The model under review builds one solid part; all positions refer to its coordinate system, in mm. Face numbers are marked on the shaded views. A direction names the side the tool comes from. Coordinates: 2 decimals unless noted, no trailing zeros. Write each loop counter-clockwise with the first axis right and the second up, starting at its lowest first coordinate (ties: lowest second). Pieces come first, ordered by that corner, then holes. Notation, with made-up numbers: M -10.75,-2.75 L 40.25,-2.75 A15 cw 40.25,6.25 Z; hole C 8,62 d7. An arc over 180 degrees is marked long. Answer as a JSON object with one key per item and string values.
```python
from build123d import *

# Parameters (mm, degrees)
SCHIZZO1_R                   = 12.5
ESTRUSIONE_ESTRUSIONE1_DEPTH = 50
TAGLIO_ESTRUSIONE1_DEPTH     = 15
TAGLIO_ESTRUSIONE3_START     = 23
TAGLIO_ESTRUSIONE3_DEPTH     = 15


with BuildPart() as part:
    # Schizzo1 → Estrusione-Estrusione1 (new body)
    with BuildSketch(Plane.XY):
        Circle(SCHIZZO1_R)
    extrude(amount=ESTRUSIONE_ESTRUSIONE1_DEPTH)

    # Schizzo2 → Taglio-Estrusione1 (cut)
    with BuildSketch(Plane.XY.offset(50)):
        Polygon((-3.175426481, 5.5), (-6.350852961, 0), (-3.175426481, -5.5), (3.175426481, -5.5), (6.350852961, 0), (3.175426481, 5.5), align=None)
    extrude(amount=-TAGLIO_ESTRUSIONE1_DEPTH, mode=Mode.SUBTRACT)

    # Schizzo3 → Taglio-Estrusione3 (cut)
    with BuildSketch(Plane(origin=(0, 0, 0), x_dir=(1, 0, 0), z_dir=(0, 1, 0)).offset(TAGLIO_ESTRUSIONE3_START)):
        with BuildLine():
            Line((3.5, -7.5), (3.5, -22.5))
            ThreePointArc((3.5, -22.5), (0, -26), (-3.5, -22.5))
            Line((-3.5, -22.5), (-3.5, -7.5))
            ThreePointArc((-3.5, -7.5), (0, -4), (3.5, -7.5))
        make_face()
    extrude(amount=-TAGLIO_ESTRUSIONE3_DEPTH, mode=Mode.SUBTRACT)


solid = part.part
```
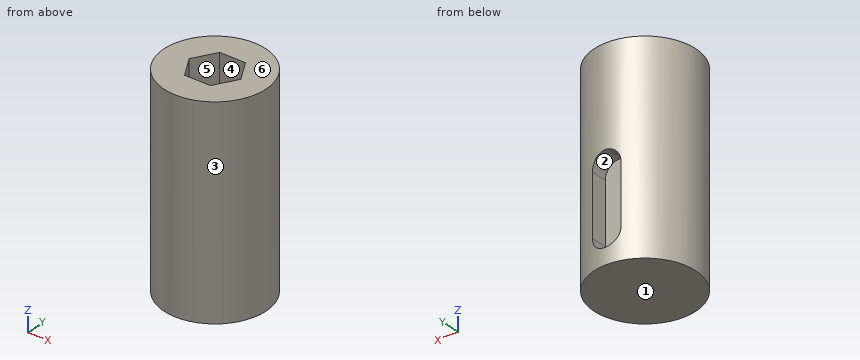
(1) Add section B-B on z = 41.5. Give the boundary of the cut face in (x, y).
Results list:
{"outline": "C 0,0 d25; hole M -6.35,0 L -3.18,-5.5 L 3.18,-5.5 L 6.35,0 L 3.18,5.5 L -3.18,5.5 Z"}
(2) Add section A-A on x = 0. Give the boundary of the cut face in (y, z), and give its area (3 significant figures).
Results list:
{"outline": "M -12.5,0 L 12.5,0 L 12.5,4 L 8,4 L 8,26 L 12.5,26 L 12.5,50 L 5.5,50 L 5.5,35 L -5.5,35 L -5.5,50 L -12.5,50 Z", "area": "986 mm²"}
(3) Add section D-D on z = 17.5. Give the boundary of the cut face in (x, y), and give its area (3 significant figures).
Results list:
{"outline": "M -3.5,8 L -3.5,12 A12.5 ccw long 3.5,12 L 3.5,8 Z", "area": "461 mm²"}
(4) Draft analysis for pull direction Y (two halves, no side actions). For the marked faces 3, 4, 5 and 6, state which applies: released by +Y, released by -Y, zero draft, split by the parting line, or undercut.
Results list:
{"face 3": "split by the parting line", "face 4": "undercut", "face 5": "undercut", "face 6": "zero draft"}
(5) Wall thickness on line 1 along Y through (x, z) = (0, 36); line 2 along Y through (x, z) = (-1.5, 36); line 3 along Z through (x, y) = (2.75, -0.25): over which ranges is each line inside the solid? List them lowest first. Write a range as from..to.
Results list:
{"line 1": "-12.5..-5.5, 5.5..12.5", "line 2": "-12.41..-5.5, 5.5..12.41", "line 3": "0..35"}
(6) Add section C-C on y = 4. Give the boundary of the cut face in (x, z), and give its area (3 significant figures).
Results list:
{"outline": "M -11.84,0 L 11.84,0 L 11.84,50 L 4.04,50 L 4.04,35 L -4.04,35 L -4.04,50 L -11.84,50 Z", "area": "1,060 mm²"}
(7) For pin 1 Ø3 at (x, z) = (-1.5, 39.5) entering from +Y; pin 2 Ø2 at (y, z) = (10.5, 13) entering from +X; pin 3 Ø5 at (x, z) = (9, 36) entering from -Y; pin 4 Ø6 at (y, z) = (-3.5, 38.5) entering from -X, all flat-tipped, find the tip position at first contact; note any pin that passes through.
Results list:
{"pin 1": "y = 12.5", "pin 2": "x = 8.12", "pin 3": "y = -10.68", "pin 4": "x = -12.49"}
(8) For the marked faces 1 and 2, list the 3-axis set-ups (+Z, -Z, +X, -X, +Y, -Y) from which the entire face can be reached by the end or side of a thin tool; tool diameter is ignored.
Results list:
{"face 1": "-Z, +X, -X, +Y, -Y", "face 2": "+Y"}
